Here's how the part is built. I have some questions about the finished solid (model axes, mm). Face numbers are marked on the shaded views. A direction names the side the tool comes from. Round coordinates to 2 decimals unless told otherwise and drop trailing zeros. Order: outer loops, then holes, each group sorted by start corner. A loop starts at its lowest first (then second) coordinate and runs counter-clockwise, first axis right, second up. Notation, with made-up numbers: (7, -10.75) - (21, -10.75) arc R34 ccw to (21, 24.25) - close; hole circle Ø4 at (43.5, 4). An arc over 180 degrees is marked (long way). Answer as a JSON object with one key per item and string values.
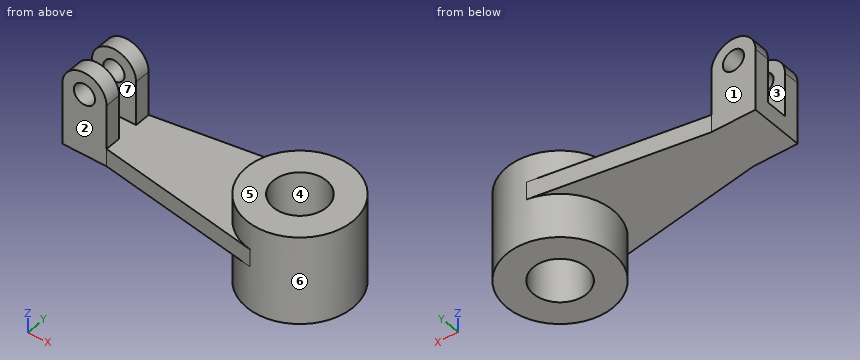
```python
from build123d import *

# Parameters (mm, degrees)
SKETCH1_R           = 30
BOSS_EXTRUDE1_DEPTH = 25
SKETCH2_R           = 15
CUT_EXTRUDE1_DEPTH  = 50
BOSS_EXTRUDE3_DEPTH = 10
SKETCH8_R           = 6
BOSS_EXTRUDE4_DEPTH = 9


with BuildPart() as part:
    # Sketch1 → Boss-Extrude1 (new body, symmetric)
    with BuildSketch(Plane.XY):
        Circle(SKETCH1_R)
    extrude(amount=BOSS_EXTRUDE1_DEPTH, both=True)

    # Sketch2 → Cut-Extrude1 (cut)
    with BuildSketch(Plane.XY.offset(25)):
        Circle(SKETCH2_R)
    extrude(amount=-CUT_EXTRUDE1_DEPTH, mode=Mode.SUBTRACT)

    # Sketch6 → Boss-Extrude3 (add)
    with BuildSketch(Plane.XY):
        with BuildLine():
            Line((-4.671688756, 29.634023084), (-97.5, 15))
            Line((-97.5, 15), (-122.5, 15))
            Line((-122.5, 15), (-122.5, -15))
            Line((-122.5, -15), (-97.5, -15))
            Line((-97.5, -15), (-4.671688756, -29.634023084))
            ThreePointArc((-4.671688756, -29.634023084), (-30, 0), (-4.671688756, 29.634023084))
        make_face()
    extrude(amount=BOSS_EXTRUDE3_DEPTH)

    # Sketch8 → Boss-Extrude4 (add)
    with BuildSketch(Plane.XZ.offset(15)):
        with BuildLine():
            Line((-122.5, 10), (-122.5, 35))
            ThreePointArc((-122.5, 35), (-110, 47.5), (-97.5, 35))
            Line((-97.5, 35), (-97.5, 10))
            Line((-97.5, 10), (-122.5, 10))
        make_face()
        with Locations((-110, 35)):
            Circle(SKETCH8_R, mode=Mode.SUBTRACT)
    boss_extrude4 = extrude(amount=-BOSS_EXTRUDE4_DEPTH)

    # Mirror1: Boss-Extrude4 across plane
    add(boss_extrude4.mirror(Plane.ZX))


solid = part.part
```
1. For P1, Ø20, axis at x = -114.5, z = 23, coming from the +Y side; P2, Ø19, axis at x = -110, z = 35, coming from the -Y side; P3, Ø12, axis at x = -53.5, y = 15.5, coming from the -Z side, each with a flat end and sliding along its axis, tell me the tip position at first contact or that it passes through.
Responses:
{"P1": "y = 15", "P2": "y = -15", "P3": "z = 0"}
2. If I drill on L1, parallel to Y at x = 0, z = 8; L2, parallel to Z at x = -110, y = -12; L3, parallel to Z at x = -16, y = 7, over which ranges is the centre line in solid material (lowest first)? Write a range as [from, to].
Responses:
{"L1": "[-30, -15], [15, 30]", "L2": "[0, 29], [41, 47.5]", "L3": "[-25, 25]"}
3. Imagine slicing it at A-A (x = 0). List the corners of the cut face in (y, z) for me, plus the area to 3 significant figures.
Responses:
{"outline": "(-30, -25) - (-15, -25) - (-15, 25) - (-30, 25) - close; (15, -25) - (30, -25) - (30, 25) - (15, 25) - close", "area": "1,500 mm2"}
4. Thinking about a two-plate mould opening in Y: for the marked faces 1, 2, 3 and 4, which applies, pulls with the +Y half, pulls with the -Y half, needs draft (parallel to the pull), parting line crosses it, or undercut?
Responses:
{"face 1": "pulls with the +Y half", "face 2": "pulls with the -Y half", "face 3": "undercut", "face 4": "undercut"}
5. Imagine slicing it at B-B (y = 0). List the corners of the cut face in (x, z) for me.
Responses:
{"outline": "(-122.5, 0) - (-30, 0) - (-30, -25) - (-15, -25) - (-15, 25) - (-30, 25) - (-30, 10) - (-122.5, 10) - close; (15, -25) - (30, -25) - (30, 25) - (15, 25) - close"}
6. Imagine slicing it at D-D (z = -18.5). List the corners of the cut face in (x, y) for me.
Responses:
{"outline": "circle Ø60 at (0, 0); hole circle Ø30 at (0, 0)"}
7. For the marked faces 5, 6 and 7, which set-ups out of +Z, -Z, +X, -X, +Y, -Y let a thin tool reach every point of the face, with its end or its side?
Responses:
{"face 5": "+Z, +X, +Y, -Y", "face 6": "none", "face 7": "+Z, -X"}
8. Imagine slicing it at C-C (y = -7.5). List the corners of the cut face in (x, z) for me.
Responses:
{"outline": "(-122.5, 0) - (-29.05, 0) - (-29.05, -25) - (-12.99, -25) - (-12.99, 25) - (-29.05, 25) - (-29.05, 10) - (-97.5, 10) - (-97.5, 35) arc R12.5 ccw to (-122.5, 35) - close; (12.99, -25) - (29.05, -25) - (29.05, 25) - (12.99, 25) - close; hole circle Ø12 at (-110, 35)"}
